Read the model definition and answer for the solid it produces. Units are mm, in the model's axes. Face numbers are marked on the shaded views. A direction names the side the tool comes from. Coordinates: 2 decimals unless noted, no trailing zeros. Order: outer loops, then holes, each group sorted by start corner. A loop starts at its lowest first (then second) coordinate and runs counter-clockwise, first axis right, second up. Notation, with made-up numbers: (12, 60.5) -> (48, 60.5) arc R23 cw to (48, 81.5) -> close; hole circle Ø7 at (86, 87.25). An arc over 180 degrees is marked (long way). Answer as a JSON object with one key per item and string values. Group by question number.
1) Given pin 1 (4.5 mm diameter, centred on x = 0, z = 10, fed in from +Y); pin 2 (1.5 mm diameter, centred on y = 0.5, z = 14, fed in from -X); pin 3 (1 mm diameter, centred on x = -15.5, z = 13.5, fed in from -Y); pin 4 (5 mm diameter, centred on x = 3.5, z = 16.5, fed in from +Y), each flat-ended and moving along its own axis, determine where each tip first touches the part or whether it passes through.
2) A tool of negligible diameter and unlimited length cuts with its end or side. For the marked faces 3 and 4, from which of +Z, -Z, +X, -X, +Y, -Y can it reach the whole face along a straight path? Write none if from no direction.
3) Consider L1, parallel to X at y = -3.25, z = 6; L2, parallel to X at y = 1.75, z = 17.25; L3, parallel to Z at x = 0, y = -2.45. Determine where each line is inside the solid, lowest interval first.
4) Section B-B on z = 10 is taken. Count the separate pieces of the cut face and the enclosed holes in it, and give its area (3 significant figures).
5) Section A-A on x = -43 is taken. Determine the outline of the cut face in (y, z), and give its area (3 significant figures).
6) Determine the mould class of the marked faces 1 and 2 for opening direction X: released by +X, released by -X, zero draft, split by the parting line, or undercut.
7) Section C-C on x = 21.5 is taken. Determine the outline of the cut face in (y, z), and give its area (3 significant figures).
from build123d import *

# Parameters (mm, degrees)
F1_DEPTH = 20
F2_R     = 1.5
F3_R     = 2
F4_DEPTH = 25


with BuildPart() as f1:
    # F0 (on Top) → F1 (new body)
    with BuildSketch(Plane.XY):
        Polygon((-40, -4), (-37, -4), (-37, 0.5), (-6, 0.5), (-6, -4), (6, -4), (6, 0.5), (37, 0.5), (37, -4), (40, -4), (46, -4), (46, -1), (40, -1), (40, 3.5), (3, 3.5), (3, -1), (0, -1), (-3, -1), (-3, 3.5), (-40, 3.5), (-40, -1), (-46, -1), (-46, -4), align=None)
    extrude(amount=F1_DEPTH)

    # F2
    f2_edges = [f1.edges().sort_by_distance(p)[0] for p in [
        (-21.5, 0.5, 0),
        (-37, -1.75, 0),
        (-6, -1.75, 0),
        (6, -1.75, 0),
        (21.5, 0.5, 0),
        (37, -1.75, 0),
        (-40, 3.5, 10),
        (-3, 3.5, 10),
        (3, 3.5, 10),
        (40, 3.5, 10),
        (-37, 0.5, 10),
        (-6, 0.5, 10),
        (6, 0.5, 10),
        (37, 0.5, 10),
    ]]
    fillet(f2_edges, radius=F2_R)

    # F3 (on face) → F4 (cut)
    with BuildSketch(Plane(origin=(0, -1, 0), x_dir=(-1, 0, 0), z_dir=(0, 1, 0))):
        with Locations((-43, 10)):
            Circle(F3_R)
        with Locations((0, 10)):
            Circle(F3_R)
        with Locations((43, 10)):
            Circle(F3_R)
    extrude(amount=-F4_DEPTH, mode=Mode.SUBTRACT)


solid = f1.part
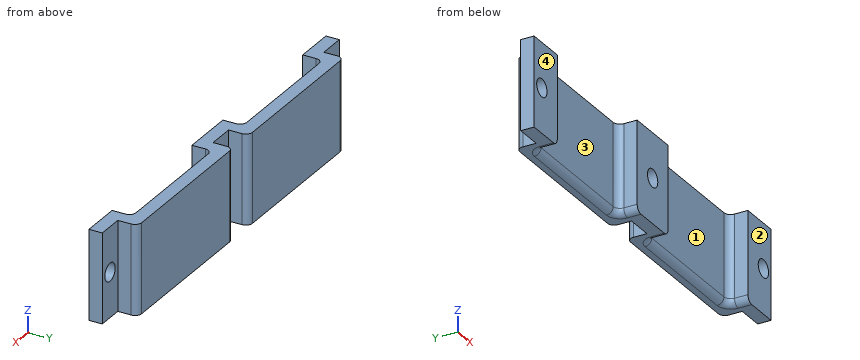
Worked answers:
{
 "1": {"pin 1": "stops at y = -1", "pin 2": "stops at x = -40", "pin 3": "stops at y = 0.5", "pin 4": "stops at y = 3.5"},
 "2": {"face 3": "+Z, -Z, -Y", "face 4": "+Z, -Z, +X, -X, -Y"},
 "3": {"L1": "x = -46 to -37, -6 to 6, 37 to 46", "L2": "x = -40 to -3, 3 to 40", "L3": "z = 0 to 8, 12 to 20"},
 "4": {"separate pieces": "4", "enclosed holes": "0", "area": "294 mm²"},
 "5": {"outline": "(-4, 0) -> (-1, 0) -> (-1, 8) -> (-4, 8) -> close; (-4, 12) -> (-1, 12) -> (-1, 20) -> (-4, 20) -> close", "area": "48.0 mm²"},
 "6": {"face 1": "undercut", "face 2": "zero draft"},
 "7": {"outline": "(0.5, 1.5) arc R1.5 ccw to (2, 0) -> (3.5, 0) -> (3.5, 20) -> (0.5, 20) -> close", "area": "59.5 mm²"}
}
